Read the model definition and answer for the solid it produces. Units are mm, in the model's axes. A direction names the side the tool comes from. Give positions to 0.01 mm unless a question says otherwise; leave off trailing zeros. Write each loop counter-clockwise with the first axis right and the second up, starting at its lowest first coordinate (ties: lowest second). Pieces come first, ordered by that corner, then holes. Notation, with made-up numbers: M 78.5,82.25 L 108.5,82.25 A27 cw 108.5,106.25 Z; hole C 17,46.25 d1. An arc over 180 degrees is marked long. Answer as CSV lines item,"result". Start each with the question number.
```python
from build123d import *

# Parameters (mm, degrees)
BOSS_EXTRUDE1_DEPTH = 15
FILLET1_RADIUS      = 7.5
FILLET1_LENGTH      = 3
FILLET2_RADIUS      = 7.5
FILLET2_LENGTH      = 3
CUT_EXTRUDE1_REACH  = 35.126
SKETCH2_R           = 2.5


with BuildPart() as part:
    # Sketch1 → Boss-Extrude1 (new body)
    with BuildSketch(Plane(origin=(0, 0, 0), x_dir=(1, 0, 0), z_dir=(0, 1, 0))):
        with BuildLine():
            Line((1, 10.602947703), (1, 23.416407865))
            Line((1, 23.416407865), (4, 23.416407865))
            Line((4, 23.416407865), (4, 15.491933385))
            ThreePointArc((4, 15.491933385), (4.479495849, 13.864954951), (5.764705882, 12.758062788))
            ThreePointArc((5.764705882, 12.758062788), (0, -14), (-5.764705882, 12.758062788))
            ThreePointArc((-5.764705882, 12.758062788), (-4.479495849, 13.864954951), (-4, 15.491933385))
            Line((-4, 15.491933385), (-4, 23.416407865))
            Line((-4, 23.416407865), (-1, 23.416407865))
            Line((-1, 23.416407865), (-1, 10.602947703))
            ThreePointArc((-1, 10.602947703), (0, -10.65), (1, 10.602947703))
        make_face()
    extrude(amount=BOSS_EXTRUDE1_DEPTH)

    # Fillet1: full round fillet: the end face becomes a half cylinder, R = half its width
    fillet1_face = Plane((-2.5, 7.5, -23.416407865), x_dir=(-1, 0, 0), z_dir=(0, 0, -1))  # on the end face: x along it, z out of the body
    fillet1_slab = fillet1_face.offset(-FILLET1_RADIUS / 2) * Box(FILLET1_LENGTH, 2 * FILLET1_RADIUS, FILLET1_RADIUS, mode=Mode.PRIVATE)  # the body's end, R deep
    fillet1_round = Plane((-2.5, 7.5, -15.916407865), x_dir=(0, 0, -1), z_dir=(-1, 0, 0)) * Cylinder(FILLET1_RADIUS, FILLET1_LENGTH, mode=Mode.PRIVATE)  # its axis R under the face
    add(fillet1_slab - fillet1_round, mode=Mode.SUBTRACT)

    # Fillet2: full round fillet: the end face becomes a half cylinder, R = half its width
    fillet2_face = Plane((2.5, 7.5, -23.416407865), x_dir=(1, 0, 0), z_dir=(0, 0, -1))  # on the end face: x along it, z out of the body
    fillet2_slab = fillet2_face.offset(-FILLET2_RADIUS / 2) * Box(FILLET2_LENGTH, 2 * FILLET2_RADIUS, FILLET2_RADIUS, mode=Mode.PRIVATE)  # the body's end, R deep
    fillet2_round = Plane((2.5, 7.5, -15.916407865), x_dir=(0, 0, -1), z_dir=(1, 0, 0)) * Cylinder(FILLET2_RADIUS, FILLET2_LENGTH, mode=Mode.PRIVATE)  # its axis R under the face
    add(fillet2_slab - fillet2_round, mode=Mode.SUBTRACT)

    # Cut-Extrude1: up to this face of the body (flat: up to its plane)
    cut_extrude1_end = Plane(part.part.faces().sort_by_distance((-4, 7.5, -18.87128147))[0])
    # Sketch2 → Cut-Extrude1 (cut, up to the picked face)
    with BuildSketch(Plane(origin=(4, 0, 0), x_dir=(0, 0, -1), z_dir=(1, 0, 0)), mode=Mode.PRIVATE) as cut_extrude1_sk1:
        with Locations(Location((15.916407865, 7.5, 0), (0, 0, 99.775597353))):
            Circle(SKETCH2_R)
    cut_extrude1_tool1 = split(extrude(cut_extrude1_sk1.sketch, amount=-CUT_EXTRUDE1_REACH, mode=Mode.PRIVATE), bisect_by=cut_extrude1_end, keep=Keep.BOTH, mode=Mode.PRIVATE)
    add(cut_extrude1_tool1.solids().sort_by(Axis((4, 7.5, -15.916408), (-1, 0, 0)))[0], mode=Mode.SUBTRACT)


solid = part.part
```
1. Find section D-D on y = 4.25. Determine the outline of the cut face in (x, z).
2. Find the intervals of material crossed by line 1 (Y direction, x = -1.75, z = -15.5); line 2 (X direction, y = 12, z = -18); line 3 (Z direction, x = 1.9, y = 7.5), in increasing order. Write a range as [from, to].
3. Find section B-B on y = 7.5. Determine the outline of the cut face in (x, z), then the cut area to 3 significant figures.
4. Given pin 1 (2 mm diameter, centred on y = 3.5, z = -16, fed in from -X); pin 2 (6.5 mm diameter, centred on y = 5.5, z = -17.5, fed in from -X); pin 3 (1 mm diameter, centred on y = 7, z = -14.5, fed in from -X), each flat-ended and moving along its own axis, determine where each tip first touches the part or whether it passes through.
5. Determine the mould class of faces 1 (the face through (-1, 7, -19)), 2 (the face through (-2.479, 7.38, -18.414)), 3 (the face through (2.521, 7.335, -23.415)), 4 (the face through (-4.493, 7.395, -13.845)) for opening direction X: +X half, -X half, draft (parallel to the pull), parting line (faces both ways), or undercut.
6. Find section C-C on z = -11. Determine the outline of the cut face in (x, y).
7. For faces 5 (the face through (4, 7, -20)), 6 (the face through (-4, 7, -14)), 7 (the face through (1, 9.1, -18.3)), 8 (the face through (-4, 7, -19)), 9 (the face through (9.4, 15, -5.5)), determine the directions among +Z, -Z, +X, -X, +Y, -Y from which every point of the face is accessible in a straight line to the end or side of a thin tool.
8. Find section A-A on z = 0. Determine the outline of the cut face in (x, y), then the cut area to 4 significant figures.
Computed:
1,outline,"M -5.76,-12.76 A3 cw -4,-15.49 L -4,-22.68 L -1,-22.68 L -1,-10.6 A10.65 cw long 1,-10.6 L 1,-22.68 L 4,-22.68 L 4,-15.49 A3 cw 5.76,-12.76 A14 ccw long Z"
2,line 1,"y = [0, 5.03], [9.97, 15]"
2,line 2,"x = [-4, -1], [1, 4]"
2,line 3,"z = [-23.42, -18.42], [-13.42, -10.48], [10.48, 13.87]"
3,outline,"M -5.76,-12.76 A3 cw -4,-15.49 L -4,-13.42 L -1,-13.42 L -1,-10.6 A10.65 cw long 1,-10.6 L 1,-13.42 L 4,-13.42 L 4,-15.49 A3 cw 5.76,-12.76 A14 ccw long Z; M -4,-23.42 L -1,-23.42 L -1,-18.42 L -4,-18.42 Z; M 1,-23.42 L 4,-23.42 L 4,-18.42 L 1,-18.42 Z"
3,area,"282 mm^2"
4,pin 1,"stops at x = -4.04"
4,pin 2,"stops at x = -4.27"
4,pin 3,"stops at x = -4.4"
5,face 1,"undercut"
5,face 2,"undercut"
5,face 3,"draft"
5,face 4,"-X half"
6,outline,"M -8.66,0 L -1,0 L -1,15 L -8.66,15 Z; M 1,0 L 8.66,0 L 8.66,15 L 1,15 Z"
7,face 5,"-Z, +X, +Y, -Y"
7,face 6,"none"
7,face 7,"-Z, +Y, -Y"
7,face 8,"-Z, -X, +Y, -Y"
7,face 9,"+Z, -Z, +X, -X, +Y"
8,outline,"M -14,0 L -10.65,0 L -10.65,15 L -14,15 Z; M 10.65,0 L 14,0 L 14,15 L 10.65,15 Z"
8,area,"100.5 mm^2"
